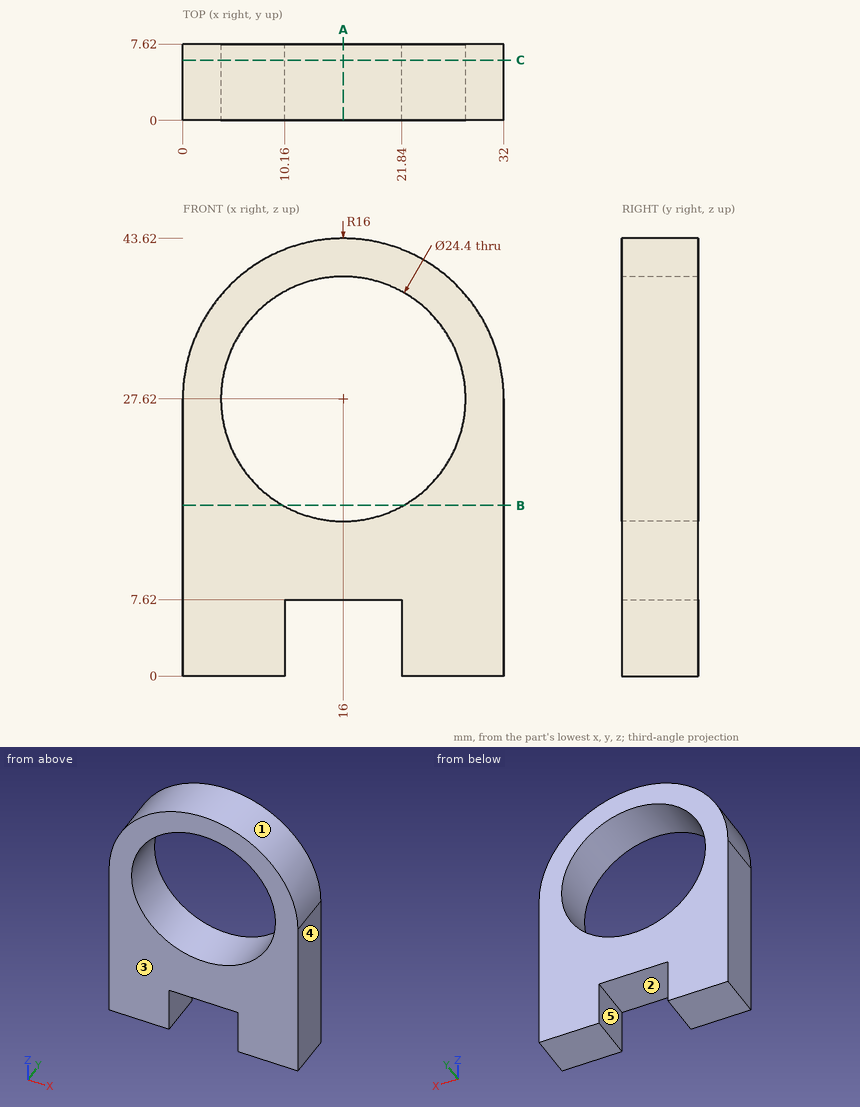
Source: three-view drawing plus pictorial views. Frame: mm from the lowest corner of the part. A direction names the side the tool comes from. Give positions to 0.01 mm unless a question says otherwise; leave off trailing zeros. Loops run counter-clockwise (first coordinate to the right, second up) from the corner with the lowest first, then second, coordinate; pieces in that order, holes last.
1) Section query A-A on x = 16. Return the cut outline in (y, z), and give its area (3 significant figures).
A:
outline: (0, 7.62) - (7.62, 7.62) - (7.62, 15.42) - (0, 15.42) - close; (0, 39.82) - (7.62, 39.82) - (7.62, 43.62) - (0, 43.62) - close
area: 88.4 mm2
2) Section query C-C on y = 6. Return the cut outline in (x, z), and give its area (3 significant figures).
A:
outline: (0, 0) - (10.16, 0) - (10.16, 7.62) - (21.84, 7.62) - (21.84, 0) - (32, 0) - (32, 27.62) arc R16 ccw to (0, 27.62) - close; hole circle Ø24.4 at (16, 27.62)
area: 729 mm2
3) Mould query, pull axis X, two halves, no side actions, for the marked faces 3, 4 and 5. Classes: released by +X, released by -X, zero draft, split by the parting line, or undercut.
A:
face 3: zero draft
face 4: released by +X
face 5: undercut
4) Contact query for flat-ended pins moving along their axis: pin 1 (4 mm diameter, centred on x = 5, y = 4.5, fed in from +Z); pin 2 (2 mm diameter, centred on x = 23.5, y = 4, fed in from +Z); pin 3 (1 mm diameter, centred on x = 6.5, z = 32.5, fed in from -Y). Output: stop coordinate, or through.
A:
pin 1: stops at z = 40.85
pin 2: stops at z = 42.24
pin 3: passes through
5) Section query B-B on z = 17. Return the cut outline in (x, y).
A:
outline: (0, 0) - (10, 0) - (10, 7.62) - (0, 7.62) - close; (22, 0) - (32, 0) - (32, 7.62) - (22, 7.62) - close
6) Line query: L1, parallel to Z at x = 16, y = 4.5; L2, parallel to X at y = 3.25, z = 4.5; L3, parallel to Z at x = 10, y = 3. Output: solid intervals per line, ascending.
A:
L1: z = 7.62 to 15.42, 39.82 to 43.62
L2: x = 0 to 10.16, 21.84 to 32
L3: z = 0 to 17, 38.24 to 42.45
7) Reachability of the marked faces 1 and 2 from +Z, -Z, +X, -X, +Y, -Y: full face, straight path, thin tool, end or side. Return the list, or none.
A:
face 1: +Z, +Y, -Y
face 2: -Z, +Y, -Y
